Answer from the drawing. Dimensions are ordinates in mm from the lowest x, y and z of the part. Give positions to 0.01 mm unless a question says otherwise; leave off trailing zeros. Write each loop counter-clockwise with the first axis right and the second up, starting at its lowest first coordinate (ties: lowest second). Pieces come first, ordered by that corner, then holes. Notation, with made-up numbers: (84, 65) -> (125, 65) arc R37 ccw to (125, 102) -> close; hole circle Ø9 at (-35, -7). An arc over 180 degrees is marked (long way). Put each result on its own line as item: value. Start each with the question number.
1) Find the intervals of material crossed by line 1 along Z through (x, y) = (37, 9); line 2 along Z through (x, y) = (22, 31.5); line 3 along Y through (x, z) = (15.5, 7), in increasing order. Write a range as from..to.
2) A flat-ended cylindrical pin translates along its axis: pin 1 Ø1.5 at (x, y) = (35.5, 32) entering from -Z. Find the tip coordinate at first contact, or state that the pin passes through.
3) A cutting plane is placed at A-A (x = 29.5). Write down the section's boundary in (y, z), then the cut area to 3 significant figures.
4) A cutting plane is placed at B-B (y = 4). Write down the section's boundary in (x, z).
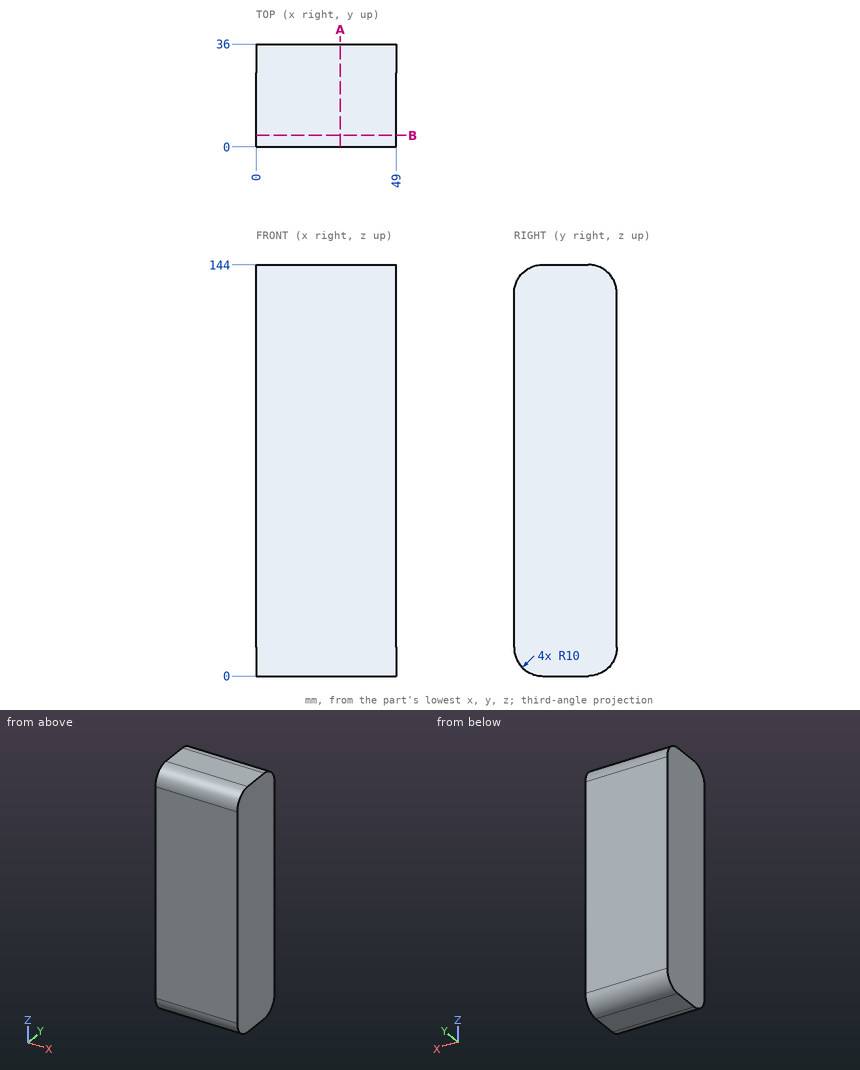
Reply:
1. line 1: z = 0.05..143.95
1. line 2: z = 1.65..142.35
1. line 3: y = 0.46..35.54
2. pin 1: stops at z = 1.49
3. outline: (0, 10) arc R10 ccw to (10, 0) -> (26, 0) arc R10 ccw to (36, 10) -> (36, 134) arc R10 ccw to (26, 144) -> (10, 144) arc R10 ccw to (0, 134) -> close
3. area: 5,100 mm2
4. outline: (0, 2) -> (49, 2) -> (49, 142) -> (0, 142) -> close
